from build123d import *

# Parameters (mm, degrees)
SKETCH1_W               = 107
SKETCH1_H               = 11
BOSS_EXTRUDE1_DEPTH     = 1.5
SKETCH3_W               = 11
SKETCH3_H               = 17
BOSS_EXTRUDE2_DEPTH     = 1.5
SKETCH4_W               = 3
SKETCH4_H               = 11
BOSS_EXTRUDE3_DEPTH     = 1.5
CUT_EXTRUDE1_DEPTH      = 69.049614253
CUT_EXTRUDE1_DEPTH_BACK = 69.049614253


with BuildPart() as part:
    # Sketch1 → Boss-Extrude1 (new, symmetric)
    with BuildSketch(Plane(origin=(0, 0, 0), x_dir=(1, 0, 0), z_dir=(0, 1, 0))):
        Rectangle(SKETCH1_W, SKETCH1_H)
    extrude(amount=BOSS_EXTRUDE1_DEPTH, both=True)

    # Sketch3 → Boss-Extrude2 (add, symmetric)
    with BuildSketch(Plane(origin=(0, 0, 0), x_dir=(1, 0, 0), z_dir=(0, 1, 0))):
        with Locations((-59, 0)):
            Rectangle(SKETCH3_W, SKETCH3_H)
        with Locations((59, 0)):
            Rectangle(SKETCH3_W, SKETCH3_H)
    extrude(amount=BOSS_EXTRUDE2_DEPTH, both=True)

    # Sketch4 → Boss-Extrude3 (add, symmetric)
    with BuildSketch(Plane(origin=(0, 0, 0), x_dir=(1, 0, 0), z_dir=(0, 1, 0))):
        with Locations((-66, 0)):
            Rectangle(SKETCH4_W, SKETCH4_H)
        with Locations((66, 0)):
            Rectangle(SKETCH4_W, SKETCH4_H)
    extrude(amount=BOSS_EXTRUDE3_DEPTH, both=True)

    # Sketch2 → Cut-Extrude1 (cut, two sides)
    with BuildSketch(Plane(origin=(0, 0, 0), x_dir=(1, 0, 0), z_dir=(0, 1, 0))) as cut_extrude1_sk:
        with BuildLine():
            Line((-67.5, 1.5), (-63.5, 1.5))
            Line((-63.5, 1.5), (-63.5, 2.85))
            Line((-63.5, 2.85), (-61.23, 2.85))
            Line((-61.23, 2.85), (-61.23, 1.5))
            Line((-61.23, 1.5), (-56.5, 1.5))
            ThreePointArc((-56.5, 1.5), (-55.792893219, 1.207106781), (-55.5, 0.5))
            Line((-55.5, 0.5), (-55.5, -0.5))
            ThreePointArc((-55.5, -0.5), (-55.792893219, -1.207106781), (-56.5, -1.5))
            Line((-56.5, -1.5), (-61.23, -1.5))
            Line((-61.23, -1.5), (-61.23, -2.85))
            Line((-61.23, -2.85), (-63.5, -2.85))
            Line((-63.5, -2.85), (-63.5, -1.5))
            Line((-63.5, -1.5), (-67.5, -1.5))
            Line((-67.5, -1.5), (-67.5, 1.5))
        make_face()
        with BuildLine():
            Line((61.23, -1.5), (56.5, -1.5))
            ThreePointArc((56.5, -1.5), (55.792893219, -1.207106781), (55.5, -0.5))
            Line((55.5, -0.5), (55.5, 0.5))
            ThreePointArc((55.5, 0.5), (55.792893219, 1.207106781), (56.5, 1.5))
            Line((56.5, 1.5), (61.23, 1.5))
            Line((61.23, 1.5), (61.23, 2.85))
            Line((61.23, 2.85), (63.5, 2.85))
            Line((63.5, 2.85), (63.5, 1.5))
            Line((63.5, 1.5), (67.5, 1.5))
            Line((67.5, 1.5), (67.5, -1.5))
            Line((67.5, -1.5), (63.5, -1.5))
            Line((63.5, -1.5), (63.5, -2.85))
            Line((63.5, -2.85), (61.23, -2.85))
            Line((61.23, -2.85), (61.23, -1.5))
        make_face()
    extrude(amount=CUT_EXTRUDE1_DEPTH, mode=Mode.SUBTRACT)
    extrude(cut_extrude1_sk.sketch, amount=-CUT_EXTRUDE1_DEPTH_BACK, mode=Mode.SUBTRACT)


solid = part.part
Part model, mm, in its own coordinate system. A direction names the side the tool comes from. Give positions to 0.01 mm unless a question says otherwise; leave off trailing zeros. Order: outer loops, then holes, each group sorted by start corner. A loop starts at its lowest first (then second) coordinate and runs counter-clockwise, first axis right, second up. Notation, with made-up numbers: (26, 40.5) - (58, 40.5) arc R18 ccw to (58, 72.5) - close; hole circle Ø9 at (51, -23.75). An arc over 180 degrees is marked (long way). Use a Markdown table: item, result.
1) Saw through at A-A on x = -45.5. List the corners of the cut face in (y, z), plus the area to 3 significant figures.
Checked values:
| item | result |
|---|---|
| outline | (-1.5, -5.5) - (1.5, -5.5) - (1.5, 5.5) - (-1.5, 5.5) - close |
| area | 33.0 mm² |
2) Flat gauge pins, fed straight in: P1, Ø1.5, axis at x = -25, y = -0.5, coming from the +Z side; P2, Ø0.9, axis at y = 0, z = 6.5, coming from the -X side; P3, Ø0.9, axis at x = 65.5, y = 0.5, coming from the -Z side. Where does each tip first touch, or does it go through?
Checked values:
| item | result |
|---|---|
| P1 | z = 5.5 |
| P2 | x = -64.5 |
| P3 | z = -5.5 |
3) 3-axis set-ups, long thin cutter, end or side, ignore diameter. For faces 5 (the flat face through (64.5, 0, 7)), 6 (the flat face through (-1, 0, 5.5)), 7 (the flat face through (-66, 0, -1.5)), 8 (the flat face through (64.5, 0, -7)): which of +Z, -Z, +X, -X, +Y, -Y reach the whole face in a straight line?
Checked values:
| item | result |
|---|---|
| face 5 | +Z, +X, +Y, -Y |
| face 6 | +Z, +Y, -Y |
| face 7 | -X, +Y, -Y |
| face 8 | -Z, +X, +Y, -Y |
4) Two-plate mould, pull along Z, no slides. Class faces 1 (the flat face through (59, 0, -1.5)), 2 (the flat face through (66, 0, 5.5)), 3 (the flat face through (-59, 0, -8.5)), 4 (the flat face through (-1, -1.5, 0)): +Z half, -Z half, draft (parallel to the pull), parting line (faces both ways), or undercut.
Checked values:
| item | result |
|---|---|
| face 1 | undercut |
| face 2 | +Z half |
| face 3 | -Z half |
| face 4 | draft |
5) Probe L1, parallel to X at y = 0.45, z = -1.75; L2, parallel to X at y = 0.9, z = 6.25; L3, parallel to Z at x = 35.5, y = -0.7. List the from-to ranges inside material, lowest first. Write a range as from..to.
Checked values:
| item | result |
|---|---|
| L1 | -67.5..-63.5, -61.23..61.23, 63.5..67.5 |
| L2 | -64.5..-53.5, 53.5..64.5 |
| L3 | -5.5..5.5 |
